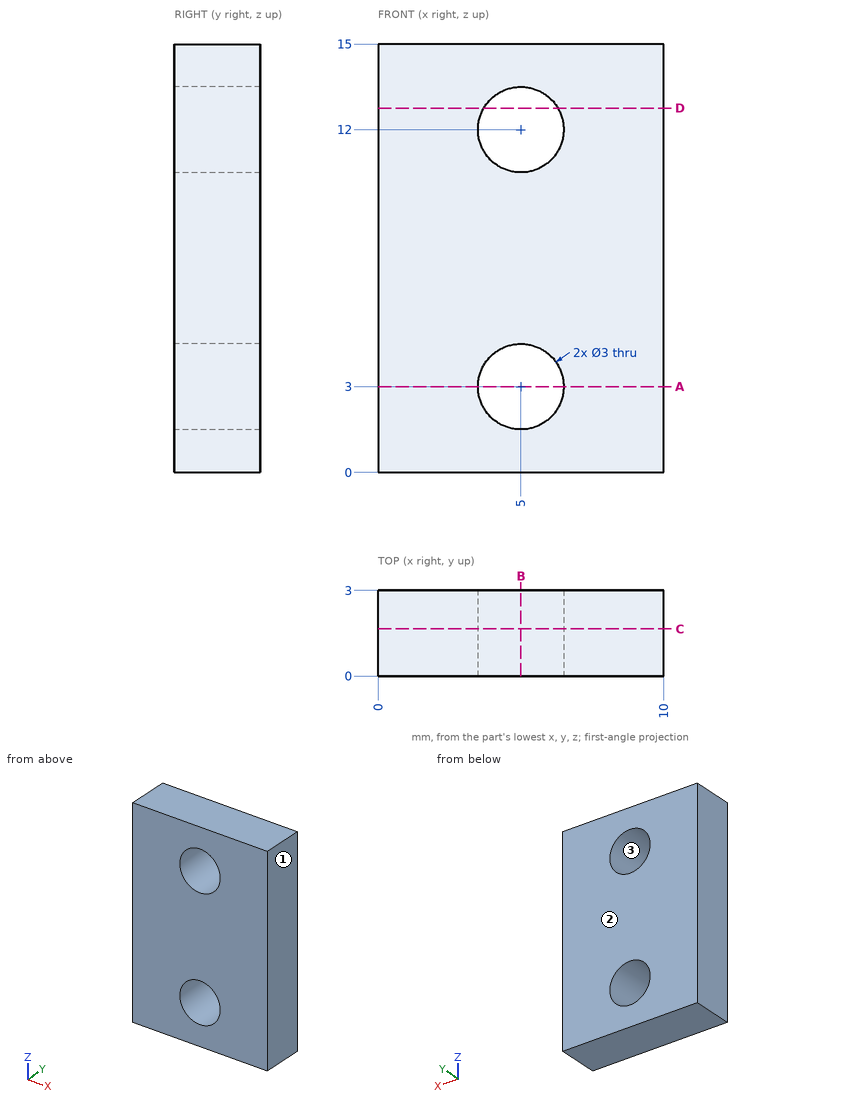
Study the drawing (mm; zero at the part's minimum x, y, z) and answer. Coordinates: 2 decimals unless noted, no trailing zeros. Loops run counter-clockwise (first coordinate to the right, second up) from the corner with the lowest first, then second, coordinate; pieces in that order, holes last. Notation, with made-up numbers: M 66,45 L 85,45 A25 cw 85,80 Z; hole C 46,-36 d1. An arc over 180 degrees is marked long. Answer in a Markdown table with one row per item.
1) Find section B-B (x = 5). Determine the outline of the cut face in (y, z), then the cut area to 3 significant figures.
Answers below:
| item | result |
|---|---|
| outline | M 0,0 L 3,0 L 3,1.5 L 0,1.5 Z; M 0,4.5 L 3,4.5 L 3,10.5 L 0,10.5 Z; M 0,13.5 L 3,13.5 L 3,15 L 0,15 Z |
| area | 27.0 mm^2 |
2) Find section D-D (z = 12.75). Determine the outline of the cut face in (x, y), then the cut area to 3 significant figures.
Answers below:
| item | result |
|---|---|
| outline | M 0,0 L 3.7,0 L 3.7,3 L 0,3 Z; M 6.3,0 L 10,0 L 10,3 L 6.3,3 Z |
| area | 22.2 mm^2 |
3) Determine the mould class of the marked faces 1, 2 and 3 for opening direction X: released by +X, released by -X, zero draft, split by the parting line, or undercut.
Answers below:
| item | result |
|---|---|
| face 1 | released by +X |
| face 2 | zero draft |
| face 3 | undercut |
4) Find the intervals of material crossed by probe 1 along Z at (x, y) = (5, 0.8); probe 2 along Z at (x, y) = (4.5, 2.1); probe 3 along X at (y, z) = (1.1, 13), in increasing order.
Answers below:
| item | result |
|---|---|
| probe 1 | 0 to 1.5, 4.5 to 10.5, 13.5 to 15 |
| probe 2 | 0 to 1.59, 4.41 to 10.59, 13.41 to 15 |
| probe 3 | 0 to 3.88, 6.12 to 10 |
5) Find section A-A (z = 3). Determine the outline of the cut face in (x, y).
Answers below:
| item | result |
|---|---|
| outline | M 0,0 L 3.5,0 L 3.5,3 L 0,3 Z; M 6.5,0 L 10,0 L 10,3 L 6.5,3 Z |
6) Find section C-C (y = 1.65). Determine the outline of the cut face in (x, z).
Answers below:
| item | result |
|---|---|
| outline | M 0,0 L 10,0 L 10,15 L 0,15 Z; hole C 5,3 d3; hole C 5,12 d3 |
